Verification items for the finished model (mm, model axes). Face numbers are marked on the shaded views. A direction names the side the tool comes from. Give positions to 0.01 mm unless a question says otherwise; leave off trailing zeros. Write each loop counter-clockwise with the first axis right and the second up, starting at its lowest first coordinate (ties: lowest second). Pieces come first, ordered by that corner, then holes.
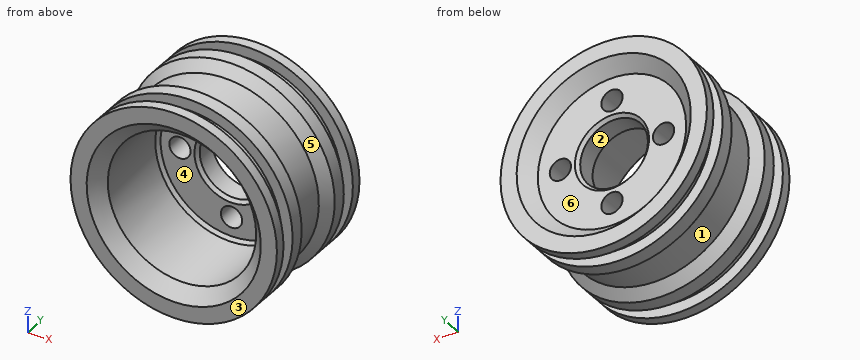
from build123d import *

# Parameters (mm, degrees)
SKETCH_1_R               = 16
EXTRUDE_1_DEPTH          = 10
SKETCH_2_W               = 1.7
SKETCH_2_H               = 2.2
SKETCH_4_R               = 11.5
CUT_EXTRUDE_1_DEPTH      = 14
SKETCH_5_R               = 5.25
CUT_EXTRUDE_2_DEPTH      = 15
CHAMFER_1_SIZE           = 2
CUT_EXTRUDE_START        = -2
SKETCH_6_R               = 11.5
SKETCH_6_R_2             = 5
CUT_EXTRUDE_3_DEPTH      = 2
CHAMFER_2_SIZE           = 2
SKETCH_8_R               = 1.65
CUT_EXTRUDE_4_DEPTH      = 10
PATTERN_CIRCULAR_1_COUNT = 4
SKETCH_7_W               = 1.5
SKETCH_7_H               = 8
CHAMFER_5_SIZE           = 1.5
CHAMFER_4_SIZE           = 0.5


with BuildPart() as part:
    # 草图1 → 凸台-拉伸1 (new, symmetric)
    with BuildSketch(Plane(origin=(0, 0, 0), x_dir=(1, 0, 0), z_dir=(0, 1, 0))):
        with Locations(Location((0, 0, 0), (0, 0, 270))):
            Circle(SKETCH_1_R)
    extrude(amount=EXTRUDE_1_DEPTH, both=True)

    # 草图2 → 切除-旋转1 (revolve, cut)
    with BuildSketch(Plane.XY, mode=Mode.PRIVATE) as cut_revolve_1_sk:
        with Locations((15.15, 7.3)):
            Rectangle(SKETCH_2_W, SKETCH_2_H)
    cut_revolve_1 = revolve(cut_revolve_1_sk.sketch.rotate(Axis((0, 8.4, 0), (0, -1, 0)), 90), axis=Axis((0, 8.4, 0), (0, -1, 0)), mode=Mode.SUBTRACT)

    # 镜向1: 切除-旋转1 across plane
    add(cut_revolve_1.mirror(Plane.ZX), mode=Mode.SUBTRACT)

    # 草图4 → 切除-拉伸1 (cut)
    with BuildSketch(Plane.XZ.offset(10)):
        with Locations(Location((0, 0, 0), (0, 0, 270))):
            Circle(SKETCH_4_R)
    extrude(amount=-CUT_EXTRUDE_1_DEPTH, mode=Mode.SUBTRACT)

    # 草图5 → 切除-拉伸2 (cut)
    with BuildSketch(Plane(origin=(0, 10, 0), x_dir=(1, 0, 0), z_dir=(0, 1, 0))):
        with Locations(Location((0, 0, 0), (0, 0, 270))):
            Circle(SKETCH_5_R)
    extrude(amount=-CUT_EXTRUDE_2_DEPTH, mode=Mode.SUBTRACT)

    # 倒角1
    chamfer_1_edges = [part.edges().sort_by_distance(p)[0] for p in [
        (0, -10, 11.5),
    ]]
    chamfer(chamfer_1_edges, length=CHAMFER_1_SIZE)

    # 草图6 → 切除-拉伸3 (cut)
    with BuildSketch(Plane(origin=(0, 10, 0), x_dir=(1, 0, 0), z_dir=(0, 1, 0)).offset(CUT_EXTRUDE_START)):
        with Locations(Location((0, 0, 0), (0, 0, 90))):
            Circle(SKETCH_6_R)
        Circle(SKETCH_6_R_2, mode=Mode.SUBTRACT)
    extrude(amount=CUT_EXTRUDE_3_DEPTH, mode=Mode.SUBTRACT)

    # 倒角2
    chamfer_2_edges = [part.edges().sort_by_distance(p)[0] for p in [
        (0, 10, 11.5),
    ]]
    chamfer(chamfer_2_edges, length=CHAMFER_2_SIZE - 0.0001)  # a hair under: the kernel refuses the full size

    # 草图8 → 切除-拉伸4 (cut)
    with BuildSketch(Plane.XZ.offset(-4)):
        with Locations(Location((-8, 0, 0), (0, 0, 270))):
            Circle(SKETCH_8_R)
    cut_extrude_4 = extrude(amount=-CUT_EXTRUDE_4_DEPTH, mode=Mode.SUBTRACT)

    # 阵列(圆周)1: 切除-拉伸4 ×4 about axis
    pattern_circular_1_axis = Axis((0, 0, 0), (0, 1, 0))
    for i in range(1, PATTERN_CIRCULAR_1_COUNT):
        add(cut_extrude_4.rotate(pattern_circular_1_axis, i * 360 / PATTERN_CIRCULAR_1_COUNT), mode=Mode.SUBTRACT)

    # 草图7 → 切除-旋转2 (revolve, cut)
    with BuildSketch(Plane(origin=(0, 0, 0), x_dir=(0, 0, -1), z_dir=(1, 0, 0))):
        with Locations((15.25, 0)):
            Rectangle(SKETCH_7_W, SKETCH_7_H)
    revolve(axis=Axis((0, 4, 0), (0, 1, 0)), mode=Mode.SUBTRACT)

    # 倒角5
    chamfer_5_edges = [part.edges().sort_by_distance(p)[0] for p in [
        (0, -4, 14.5),
        (0, 4, 14.5),
    ]]
    chamfer(chamfer_5_edges, length=CHAMFER_5_SIZE - 0.0001)  # a hair under: the kernel refuses the full size

    # 倒角4
    chamfer_4_edges = [part.edges().sort_by_distance(p)[0] for p in [
        (0, 4, 11.5),
        (0, 4, -5.25),
        (0, 8, -5.25),
    ]]
    chamfer(chamfer_4_edges, length=CHAMFER_4_SIZE)


solid = part.part
Item 1: Set-up check for the marked faces 4, 5 and 6: record each of +Z, -Z, +X, -X, +Y, -Y from which the full face is reachable in a straight line by a thin tool's end or side.
Answer key:
face 4: -Y
face 5: none
face 6: +Y
Item 2: Sectioned sample at A-A on x = 0. State how many separate pieces and enclosed holes the cut face has, then the cut area to 3 significant figures.
Answer key:
separate pieces: 4
enclosed holes: 0
area: 161 mm2
Item 3: Release check for a two-part mould opening along Y. For the marked faces 1, 2 and 3 record: released by +Y, released by -Y, zero draft, split by the parting line, or undercut.
Answer key:
face 1: undercut
face 2: zero draft
face 3: released by -Y
Item 4: Scan lines: line 1 along X through (y, z) = (5.4, 0); line 2 along X through (y, z) = (7.05, 0); line 3 along X through (y, z) = (-1.25, 0). Record each from-to range of solid material in increasing order.
Answer key:
line 1: x = -16 to -9.65, -6.35 to -5.25, 5.25 to 6.35, 9.65 to 16
line 2: x = -14.3 to -9.65, -6.35 to -5.25, 5.25 to 6.35, 9.65 to 14.3
line 3: x = -14.5 to -11.5, 11.5 to 14.5
Item 5: Depth check by flat-ended pin: pin 1 (9.5 mm diameter, centred on x = -3, z = 3.5, fed in from +Y); pin 2 (2 mm diameter, centred on x = 3, y = 0, fed in from +Z); pin 3 (5 mm diameter, centred on x = -8, z = 5.5, fed in from -Y). Enter the tip coordinate at first touch or a pass-through.
Answer key:
pin 1: stops at y = 8
pin 2: stops at z = 14.36
pin 3: stops at y = -8.71
Item 6: Sectioned sample at B-B on y = -7.25. Record the cut outline in (x, z), then the cut area to 3 significant figures.
Answer key:
outline: circle Ø28.6 at (0, 0); hole circle Ø23 at (0, 0)
area: 227 mm2
Item 7: Sectioned sample at C-C on y = 2. Record the cut outline in (x, z).
Answer key:
outline: circle Ø29 at (0, 0); hole circle Ø23 at (0, 0)
